Answer from the drawing. Dimensions are ordinates in mm from the lowest x, y and z of the part. A direction names the side the tool comes from. Round coordinates to 2 decimals unless told otherwise and drop trailing zeros. Order: outer loops, then holes, each group sorted by start corner. A loop starts at its lowest first (then second) coordinate and runs counter-clockwise, first axis right, second up. Notation, with made-up numbers: M 21,-31.75 L 54,-31.75 A28 ccw 54,-9.75 Z; hole C 15.25,-32.75 d6. An arc over 180 degrees is marked long. Use one line per item in the form item = value. Start each with the question number.
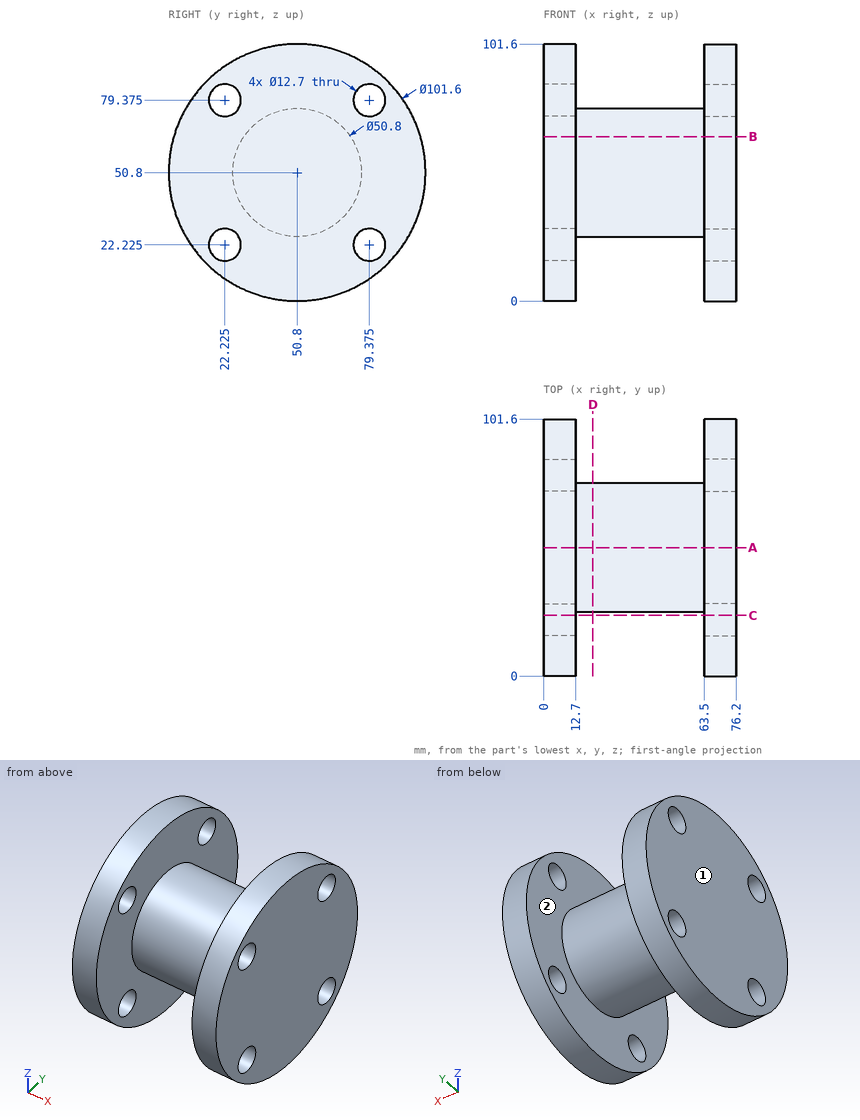
Item 1: Find the intervals of material crossed by L1, parallel to X at y = 5, z = 32; L2, parallel to Z at x = 8.5, y = 84; L3, parallel to Z at x = 71, y = 82, in increasing order. Write a range as [from, to].
Item 2: A tool of negligible diameter and unlimited length cuts with its end or side. For the marked faces 1 and 2, from which of +Z, -Z, +X, -X, +Y, -Y can it reach the whole face along a straight path? Write none if from no direction.
Item 3: Section B-B (z = 65) is taken. Write down the section's boundary in (x, y) (3 decimals), and give its area (3 significant figures).
Item 4: Given P1, Ø7.5, axis at y = 79.375, z = 79.375, coming from the +X side; P2, Ø6, axis at x = 13.5, y = 48.5, coming from the -Z side; P3, Ø3, axis at x = 47.5, y = 66, coming from the -Z side; P4, Ø12, axis at x = 53, y = 68.5, coming from the -Z side, each flat-ended and moving along its own axis, determine where each tip first touches the part or whether it passes through.
Item 5: Section C-C (y = 24) is taken. Write down the section's boundary in (x, z).
Item 6: Section D-D (x = 19.5) is taken. Write down the section's boundary in (y, z).
Item 7: Section A-A (y = 50.8) is taken. Write down the section's boundary in (x, z), and give its area (3 significant figures).
The answers:
q1.L1 = [0, 12.7], [63.5, 76.2]
q1.L2 = [12.35, 17.87], [26.58, 75.02], [83.73, 89.25]
q1.L3 = [10.71, 16.44], [28.01, 73.59], [85.16, 90.89]
q2.face_1 = +Z, -Z, -X, +Y, -Y
q2.face_2 = none
q3.outline = M 0,2.025 L 12.7,2.025 L 12.7,29.74 L 63.5,29.74 L 63.5,2.025 L 76.2,2.025 L 76.2,99.575 L 63.5,99.575 L 63.5,71.86 L 12.7,71.86 L 12.7,99.575 L 0,99.575 Z
q3.area = 4,620 mm²
q4.P1 = through
q4.P2 = 0
q4.P3 = 29.41
q4.P4 = 28.26
q5.outline = M 0,7.64 L 12.7,7.64 L 12.7,16.13 L 0,16.13 Z; M 0,28.32 L 12.7,28.32 L 12.7,73.28 L 0,73.28 Z; M 0,85.47 L 12.7,85.47 L 12.7,93.96 L 0,93.96 Z; M 63.5,7.64 L 76.2,7.64 L 76.2,16.13 L 63.5,16.13 Z; M 63.5,28.32 L 76.2,28.32 L 76.2,73.28 L 63.5,73.28 Z; M 63.5,85.47 L 76.2,85.47 L 76.2,93.96 L 63.5,93.96 Z
q6.outline = C 50.8,50.8 d50.8
q7.outline = M 0,0 L 12.7,0 L 12.7,25.4 L 63.5,25.4 L 63.5,0 L 76.2,0 L 76.2,101.6 L 63.5,101.6 L 63.5,76.2 L 12.7,76.2 L 12.7,101.6 L 0,101.6 Z
q7.area = 5,160 mm²
